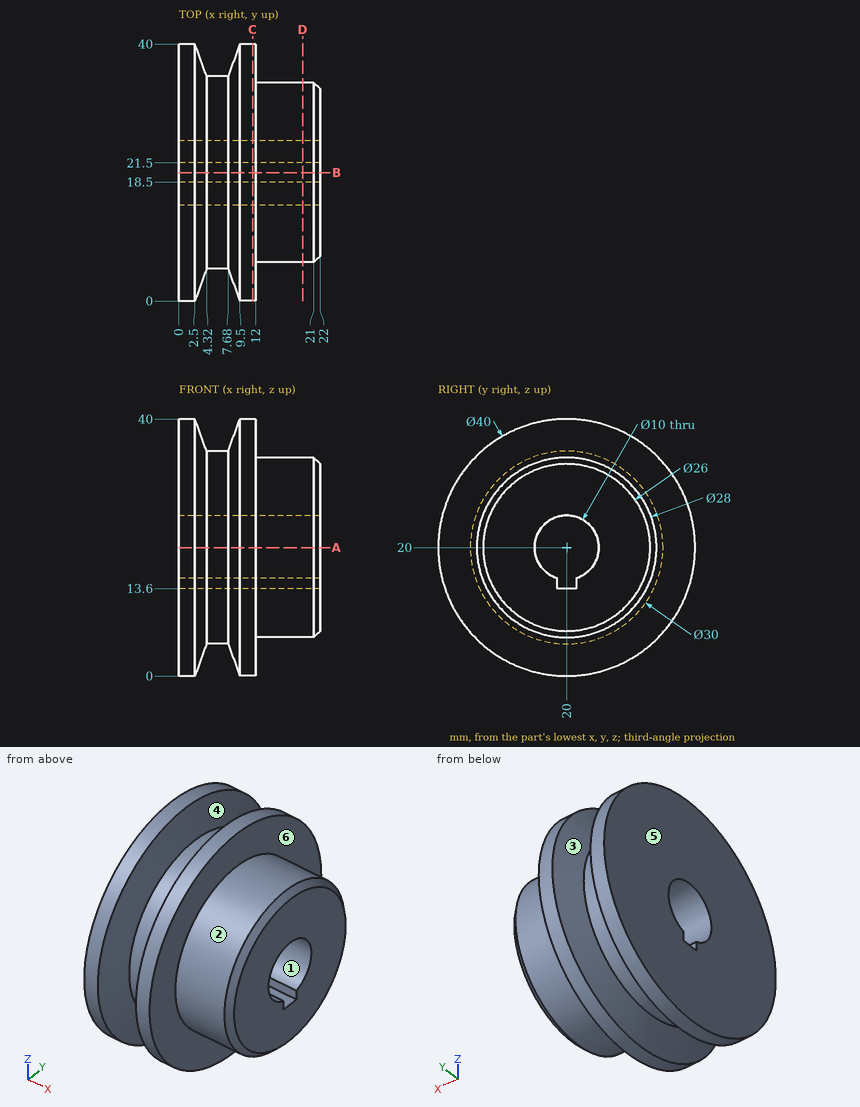
Study the drawing (mm; zero at the part's minimum x, y, z) and answer. A direction names the side the tool comes from. Coordinates: 2 decimals unless noted, no trailing zeros. Write each loop counter-clockwise with the first axis right and the second up, starting at its lowest first coordinate (ties: lowest second). Pieces come first, ordered by that corner, then holes. Notation, with made-up numbers: M 65,48 L 85,48 A9 ccw 85,56 Z; hole C 23.25,16.5 d2. An arc over 180 degrees is marked long. Use a Markdown table: item, result. Add a question column.
1. Which of the six approach directions +Z, -Z, +X, -X, +Y, -Y give full straight-line access (tool end or side, diameter ignored) to the marked faces 1 and 2?
2. Section A-A (z = 20) is taken. Give the vertices of the cut face in (x, y).
3. Section C-C (x = 11.5) is taken. Give the vertices of the cut face in (y, z).
4. For a pull along X with two mould halves and no side action, classify the marked faces 3, 4, 5 and 6 as +X half, -X half, draft (parallel to the pull), parting line (faces both ways), or undercut.
5. Straight lines are drawn through the part: line 1 along X through (y, z) = (19, 38); line 2 along Y through (x, z) = (20.5, 22); line 3 along X through (y, z) = (26, 36). For each, find the intervals that lie inside material, in ascending order. Write a range as [from, to].
6. Given P1, Ø8, axis at x = 8.5, z = 27.5, coming from the +Y side; P2, Ø6, axis at x = 15.5, y = 16, coming from the -Z side; P3, Ø3.5, axis at x = 16.5, y = 19.5, coming from the +Z side, each flat-ended and moving along its own axis, determine where each tip first touches the part or whether it passes through.
7. Section B-B (y = 20) is taken. Give the vertices of the cut face in (x, z).
8. Section D-D (x = 19.25) is taken. Give the vertices of the cut face in (y, z).
Data:
| question | item | result |
|---|---|---|
| 1 | face 1 | +X, -X |
| 1 | face 2 | +X |
| 2 | outline | M 0,0 L 2.5,0 L 4.32,5 L 7.68,5 L 9.5,0 L 12,0 L 12,6 L 21,6 L 22,7 L 22,15 L 0,15 Z; M 0,25 L 22,25 L 22,33 L 21,34 L 12,34 L 12,40 L 9.5,40 L 7.68,35 L 4.32,35 L 2.5,40 L 0,40 Z |
| 3 | outline | C 20,20 d40; hole M 18.5,13.6 L 21.5,13.6 L 21.5,15.23 A5 ccw long 18.5,15.23 Z |
| 4 | face 3 | undercut |
| 4 | face 4 | undercut |
| 4 | face 5 | -X half |
| 4 | face 6 | +X half |
| 5 | line 1 | x = [0, 3.22], [8.78, 12] |
| 5 | line 2 | y = [6.14, 15.42], [24.58, 33.86] |
| 5 | line 3 | x = [0, 3.56], [8.44, 12] |
| 6 | P1 | stops at y = 39.67 |
| 6 | P2 | stops at z = 6.04 |
| 6 | P3 | stops at z = 34 |
| 7 | outline | M 0,0 L 2.5,0 L 4.32,5 L 7.68,5 L 9.5,0 L 12,0 L 12,6 L 21,6 L 22,7 L 22,13.6 L 0,13.6 Z; M 0,25 L 22,25 L 22,33 L 21,34 L 12,34 L 12,40 L 9.5,40 L 7.68,35 L 4.32,35 L 2.5,40 L 0,40 Z |
| 8 | outline | C 20,20 d28; hole M 18.5,13.6 L 21.5,13.6 L 21.5,15.23 A5 ccw long 18.5,15.23 Z |
